```python
from build123d import *

# Parameters (mm, degrees)
F1_DEPTH = 45.72
F2_W     = 101.6
F2_H     = 35.6616
F3_DEPTH = 63.5
F4_W     = 38.2081334517
F4_H     = 25.4
F5_DEPTH = 30.48
F6_W     = 19.9782385411
F6_H     = 25.4
F7_DEPTH = 50.8


with BuildPart() as f1:
    # F0 (on Top) → F1 (new body)
    with BuildSketch(Plane.XY):
        Polygon((0, -119.299590295), (-50.8, -119.299590295), (-76.2, -119.299590295), (-62.2840667259, -194.2181247248), (62.2840667259, -194.2181247248), (76.2, -119.299590295), (50.8, -119.299590295), align=None)
    extrude(amount=F1_DEPTH)

    # F2 (on face) → F3 (cut)
    with BuildSketch(Plane(origin=(0, -119.299590295, 0), x_dir=(-1, 0, 0), z_dir=(0, 1, 0))):
        with Locations((0, 22.9217616037)):
            Rectangle(F2_W, F2_H)
    extrude(amount=-F3_DEPTH, mode=Mode.SUBTRACT)

    # F4 (on face) → F5 (join)
    with BuildSketch(Plane.XZ.offset(194.2181247248)):
        with Locations((1.7259e-06, 22.86)):
            Rectangle(F4_W, F4_H)
    extrude(amount=F5_DEPTH)

    # F6 (on face) → F7 (join)
    with BuildSketch(Plane(origin=(-19.104065, 0, 0), x_dir=(0, -1, 0), z_dir=(-1, 0, 0))):
        with Locations((214.7090054543, 22.86)):
            Rectangle(F6_W, F6_H)
        Polygon((204.7198861837, 10.16), (204.7198861837, 0), (331.7198861837, 0), (331.7198861837, 45.72), (204.7198861837, 45.72), (204.7198861837, 35.56), (224.6981247248, 35.56), (224.6981247248, 10.16), align=None)
    extrude(amount=F7_DEPTH)

    # F8: F1 across plane


with BuildPart() as f1_1:
    add(f1.part)
    add(f1.part.mirror(Plane.YZ))


solid = f1_1.part
```
Here's how the part is built. I have some questions about the finished solid (model axes, mm). A direction names the side the tool comes from. Give positions to 0.01 mm unless a question says otherwise; leave off trailing zeros. Order: outer loops, then holes, each group sorted by start corner. A loop starts at its lowest first (then second) coordinate and runs counter-clockwise, first axis right, second up. Notation, with made-up numbers: (69.5, -11.5) - (82.5, -11.5) arc R18 ccw to (82.5, 0.5) - close; hole circle Ø8 at (-7, 8.5). An arc over 180 degrees is marked (long way). Answer as a JSON object with one key per item and string values. Group by question number.
Item 1: If we section it at C-C on y = -222: Please give me the cut outline in (x, z), and give its area (3 significant figures).
Item 2: If we section it at B-B on x = 25: Please give me the cut outline in (y, z).
Item 3: If we section it at D-D on z = 30.5: Please give me the cut outline in (x, y), and give its area (3 significant figures).
Item 4: Please list where these lines run through material, in increasing order: probe 1 along Z at (x, y) = (17, -157); probe 2 along Y at (x, z) = (27.5, 37); probe 3 along X at (y, z) = (-265, 11.5).
Item 5: If we mould it in two halves opening along X, with no side actions, what happens to faces 6 (the flat face through (44, -204.72, 23)), 7 (the flat face through (-50.8, -151, 23)), 8 (the flat face through (69.145, -157.283, 22.54))? For each: pulls with the +X half, pulls with the -X half, needs draft (parallel to the pull), parting line crosses it, or undercut.
Item 6: Which directions (+Z, -Z, +X, -X, +Y, -Y) give clear straight access to the entire face, cutting with the end or side of a thin tool? Please do faces 1 (the flat face through (0, -224.698, 23)), 2 (the flat face through (1, -182.8, 23)), 3 (the flat face through (0, -209, 35.56)), 4 (the flat face through (-19.104, -199, 23)), 5 (the flat face through (-69.904, -267, 23)).
Item 7: For P1, Ø10, axis at y = -154, z = 27.5, coming from the -X side; P2, Ø6, axis at x = -54, y = -268, coming from the -Z side; P3, Ø6, axis at y = -210.5, z = 40.5, coming from the -X side; P4, Ø24.5, axis at x = -4, y = -210.5, coming from the +Z side, each with a flat end and sliding along its axis, tell me the tip position at first contact or that it passes through.
Item 8: If we section it at A-A on y = -244: Please give me the cut outline in (x, z), and give its area (3 significant figures).
Result set:
{
 "1": {"outline": "(-69.9, 0) - (-19.1, 0) - (-19.1, 10.16) - (19.1, 10.16) - (19.1, 0) - (69.9, 0) - (69.9, 45.72) - (19.1, 45.72) - (19.1, 35.56) - (-19.1, 35.56) - (-19.1, 45.72) - (-69.9, 45.72) - close", "area": "5,620 mm²"},
 "2": {"outline": "(-331.72, 0) - (-204.72, 0) - (-204.72, 45.72) - (-331.72, 45.72) - close; (-194.22, 0) - (-119.3, 0) - (-119.3, 5.09) - (-182.8, 5.09) - (-182.8, 40.75) - (-119.3, 40.75) - (-119.3, 45.72) - (-194.22, 45.72) - close"},
 "3": {"outline": "(-76.2, -119.3) - (-62.28, -194.22) - (-19.1, -194.22) - (-19.1, -204.72) - (-69.9, -204.72) - (-69.9, -331.72) - (-19.1, -331.72) - (-19.1, -224.7) - (19.1, -224.7) - (19.1, -331.72) - (69.9, -331.72) - (69.9, -204.72) - (19.1, -204.72) - (19.1, -194.22) - (62.28, -194.22) - (76.2, -119.3) - (50.8, -119.3) - (50.8, -182.8) - (-50.8, -182.8) - (-50.8, -119.3) - close", "area": "18,000 mm²"},
 "4": {"probe 1": "0 to 5.09, 40.75 to 45.72", "probe 2": "-331.72 to -204.72, -194.22 to -182.8", "probe 3": "-69.9 to -19.1, 19.1 to 69.9"},
 "5": {"face 6": "needs draft", "face 7": "undercut", "face 8": "pulls with the +X half"},
 "6": {"face 1": "+Z, -Z, -Y", "face 2": "+Y", "face 3": "+Z, -Y", "face 4": "+Z, -Z, -X", "face 5": "+Z, -Z, -X, -Y"},
 "7": {"P1": "x = -70.68", "P2": "z = 0", "P3": "x = -69.9", "P4": "z = 35.56"},
 "8": {"outline": "(-69.9, 0) - (-19.1, 0) - (-19.1, 45.72) - (-69.9, 45.72) - close; (19.1, 0) - (69.9, 0) - (69.9, 45.72) - (19.1, 45.72) - close", "area": "4,650 mm²"}
}
